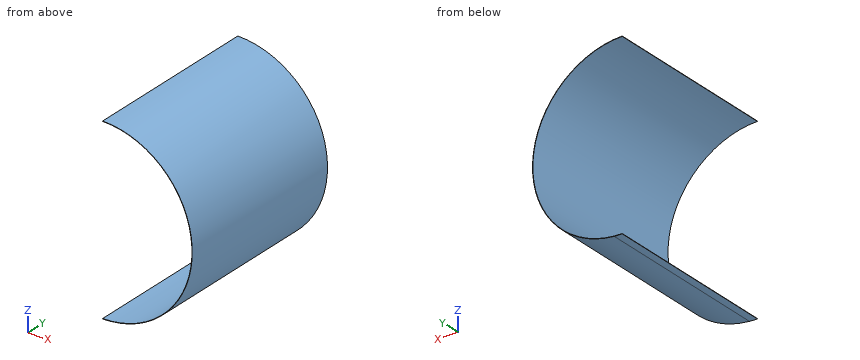
from build123d import *

# Parameters (mm, degrees)
SKETCH1_W          = 10000
SKETCH1_H          = 760
BASE_FLANGE1_DEPTH = 1.5
HEM2_START         = -380
HEM2_DEPTH         = 760
HEM2_2_DEPTH       = 760
SKETCH17_W         = 11222.895029189
SKETCH17_H         = 1018.315302658
CUT_EXTRUDE2_DEPTH = 5115.438605556


# Read off the part's stored shape, not the designer's step: Hem2
# Sheet-metal steps are written as plain solids
with BuildPart() as part:
    # Sketch1 → Base-Flange1 (new body)
    with BuildSketch(Plane.XY):
        Rectangle(SKETCH1_W, SKETCH1_H)
    extrude(amount=-BASE_FLANGE1_DEPTH)

    # Hem2 outline → Hem2 (cut)
    with BuildSketch(Plane(origin=(0, 0, 0), x_dir=(1, 0, 0), z_dir=(0, 1, 0)).offset(HEM2_START)):
        with BuildLine():
            ThreePointArc((4618.5, 1.5), (4635.415229824, 1.124815513), (4652.297189232, 0))
            Line((4652.297189232, 0), (5000, 0))
            Line((5000, 0), (5000, 1.5))
            Line((5000, 1.5), (4618.5, 1.5))
        make_face()
    extrude(amount=HEM2_DEPTH, mode=Mode.SUBTRACT)

    # Hem2 2 outline → Hem2 2 (add)
    with BuildSketch(Plane(origin=(0, 0, 0), x_dir=(1, 0, 0), z_dir=(0, 1, 0)).offset(HEM2_START)):
        with BuildLine():
            Line((4618.5, -760), (4618.5, -761.5))
            ThreePointArc((4618.5, -761.5), (4999.624815513, -396.915229824), (4652.297189232, 0))
            Line((4652.297189232, 0), (4618.5, 0))
            ThreePointArc((4618.5, 0), (4998.5, -380), (4618.5, -760))
        make_face()
    extrude(amount=HEM2_2_DEPTH)

    # Sketch17 → Cut-Extrude2 (cut, through all)
    with BuildSketch(Plane.XZ.offset(380)):
        with Locations((-992.947514595, -509.157651329)):
            Rectangle(SKETCH17_W, SKETCH17_H)
    extrude(amount=-CUT_EXTRUDE2_DEPTH, mode=Mode.SUBTRACT)


solid = part.part
Read the model definition and answer for the solid it produces. Units are mm, in the model's axes. Coordinates: 2 decimals unless noted, no trailing zeros. Order: outer loops, then holes, each group sorted by start corner. A loop starts at its lowest first (then second) coordinate and runs counter-clockwise, first axis right, second up. Notation, with made-up numbers: (65.25, 69) -> (97.25, 69) arc R13 ccw to (97.25, 77) -> close; hole circle Ø4 at (48, 11). An arc over 180 degrees is marked (long way). Answer as a JSON object with one key per item and string values.
1) Each of these flat-tipped pins is pushed along its axis until it touches: pin 1 (2 mm diameter, centred on y = -50.5, z = 341, fed in from +X); pin 2 (5 mm diameter, centred on x = 4938.5, y = 110.5, fed in from -Z); pin 3 (6 mm diameter, centred on y = 240.5, z = 553.5, fed in from +X). Where does it stop, or does it pass through?
Model answer:
{"pin 1": "stops at x = 4998.1", "pin 2": "stops at z = 168.49", "pin 3": "stops at x = 4959.78"}
2) A cutting plane is placed at D-D, the plane x = 4826.5. Determine the outline of the cut face in (y, z), plus the area to 3 significant figures.
Model answer:
{"outline": "(-380, 60.19) -> (380, 60.19) -> (380, 61.98) -> (-380, 61.98) -> close; (-380, 698.02) -> (380, 698.02) -> (380, 699.81) -> (-380, 699.81) -> close", "area": "2,720 mm²"}
3) A cutting plane is placed at C-C, the plane z = 380. Determine the outline of the cut face in (x, y).
Model answer:
{"outline": "(4998.5, -380) -> (5000, -380) -> (5000, 380) -> (4998.5, 380) -> close"}
4) A cutting plane is placed at B-B, the plane y = -115. Determine the outline of the cut face in (x, z), plus the area to 3 significant figures.
Model answer:
{"outline": "(4618.5, -1.5) arc R381.5 ccw to (4618.5, 761.5) -> (4618.5, 760) arc R380 cw to (4618.5, 0) -> close", "area": "1,790 mm²"}
5) Consider line 1 along Z through (x, y) = (4947.5, -27.5); line 2 along Z through (x, y) = (4900.5, 289.5); line 3 along X through (y, z) = (-38.5, 313). Determine where each line is inside the solid, lowest interval first. Write a range as from..to.
Model answer:
{"line 1": "z = 186.86..189.84, 570.16..573.14", "line 2": "z = 123.06..125.29, 634.71..636.94", "line 3": "x = 4992.55..4994.07"}
